from build123d import *

# Parameters (mm, degrees)
F1_DEPTH  = 459.486
F2_T      = -0.762
F5_D      = 5.2197
F5_DEPTH  = 0.762
F5_TIP    = 1.5681560866
F6_D      = 5.2197
F8_D      = 49.022
F10_D     = 17.4625
F13_D     = 5.2197
F13_DEPTH = 0.762
F13_TIP   = 1.5681560866


# Not quite as in the source:
# - a length typed as a fraction of an inch, garbled in the dataset ("3 / 203.2 mm" for 3/8 in), is restored


with BuildPart() as f1:
    # F0 (on Top) → F1 (new body)
    with BuildSketch(Plane.XY):
        Polygon((0, 360.045), (-512.445, 360.045), (-512.445, -360.045), (0, -360.045), (0, 0), align=None)
        Polygon((512.445, 360.045), (0, 360.045), (0, 0), (0, -360.045), (512.445, -360.045), align=None)
    extrude(amount=F1_DEPTH)

    # F2
    f2_openings = [f1.faces().sort_by_distance(p)[0] for p in [
        (0, 0, 459.486),
    ]]
    offset(amount=F2_T, openings=f2_openings)

    # F5
    with Locations(Plane.XZ.offset(360.045)):
        with Locations((-431.8, 415.036), (-215.9, 415.036), (0, 415.036), (215.9, 415.036), (431.8, 415.036)):
            Hole(F5_D / 2, depth=F5_DEPTH)
            with Locations((0, 0, -(F5_DEPTH + F5_TIP / 2))):  # 118° drill point
                Cone(0, F5_D / 2, F5_TIP, mode=Mode.SUBTRACT)

    # F6 (through all)
    with Locations(Plane.YZ.offset(512.445)):
        with Locations((-304.8, 415.036), (-101.6, 415.036), (101.6, 415.036), (304.8, 415.036)):
            Hole(F6_D / 2)

    # F8 (through all)
    with Locations(Plane.XY.offset(0.762)):
        with Locations((-371.475, -193.675)):
            Hole(F8_D / 2)

    # F10 (through all)
    with Locations(Plane.XY.offset(0.762)):
        with Locations((-485.775, 333.375), (-485.775, -333.375), (485.775, -333.375), (485.775, 333.375)):
            Hole(F10_D / 2)

    # F13
    with Locations(Plane(origin=(0, 360.045, 0), x_dir=(-1, 0, 0), z_dir=(0, 1, 0))):
        with Locations((-419.1, 445.1985), (-279.4, 445.1985), (-139.7, 445.1985), (0, 445.1985), (139.7, 445.1985), (279.4, 445.1985), (419.1, 445.1985)):
            Hole(F13_D / 2, depth=F13_DEPTH)
            with Locations((0, 0, -(F13_DEPTH + F13_TIP / 2))):  # 118° drill point
                Cone(0, F13_D / 2, F13_TIP, mode=Mode.SUBTRACT)


solid = f1.part
Work out the finished part from the listing and answer in its coordinate system (mm). A direction names the side the tool comes from. Round coordinates to 2 decimals unless told otherwise and drop trailing zeros. Loops run counter-clockwise (first coordinate to the right, second up) from the corner with the lowest first, then second, coordinate; pieces in that order, holes last. Notation, with made-up numbers: (84, 74.25) - (89, 74.25) arc R23 cw to (89, 112.25) - close; hole circle Ø3 at (19.25, -2). An arc over 180 degrees is marked (long way). Use one line per item in the form item = value. Start each with the question number.
(1) Find section C-C on z = 190. Determine the outline of the cut face in (x, y) (3 decimals), and give its area (3 significant figures).
(2) Find section B-B on x = 32.5. Determine the outline of the cut face in (y, z) (3 decimals), and give its area (3 significant figures).
(3) Consider line 1 (X direction, y = 194.5, z = 76.5) (3 decimals); line 2 (Y direction, x = -450, z = 439.5) (3 decimals); line 3 (Z direction, x = 469, y = 317). Determine where each line is inside the solid, lowest interval first.
(4) Which of the six approach directions +Z, -Z, +X, -X, +Y, -Y give full straight-line access (tool end or side, diameter ignored) to faces 5 (the face through (7, 360.045, 227)), 6 (the face through (-511.683, 5, 227))?
(5) Determine the mould class of faces 1 (the face through (512.445, -5, 227)), 2 (the face through (-7, 5, 0)), 3 (the face through (-512.445, 5, 227)), 4 (the face through (-7, 5, 0.762)) for opening direction X: +X half, -X half, draft (parallel to the pull), parting line (faces both ways), or undercut.
(6) Find section A-A on y = 9. Determine the outline of the cut face in (x, z) (3 decimals).
(7) Flat-ended cylindrical pins translate along their axes: P1, Ø7, axis at y = -304.8, z = 415.036, coming from the +X side (3 decimals); P2, Ø22.5, axis at x = -485.775, y = 333.375, coming from the +Z side; P3, Ø3, axis at x = -215.9, z = 415.036, coming from the -Y side. Find the tip coordinate at first contact, or state that the pin passes through.
Answer list:
q1.outline = (-512.445, -360.045) - (512.445, -360.045) - (512.445, 360.045) - (-512.445, 360.045) - close; hole (-511.683, -359.283) - (511.683, -359.283) - (511.683, 359.283) - (-511.683, 359.283) - close
q1.area = 2,660 mm^2
q2.outline = (-360.045, 0) - (360.045, 0) - (360.045, 459.486) - (359.283, 459.486) - (359.283, 0.762) - (-359.283, 0.762) - (-359.283, 459.486) - (-360.045, 459.486) - close
q2.area = 1,250 mm^2
q3.line_1 = -512.445 to -511.683, 511.683 to 512.445
q3.line_2 = -360.045 to -359.283, 359.283 to 360.045
q3.line_3 = 0 to 0.76
q4.face_5 = +Z, -Z, +X, -X, +Y
q4.face_6 = +Z
q5.face_1 = +X half
q5.face_2 = draft
q5.face_3 = -X half
q5.face_4 = undercut
q6.outline = (-512.445, 0) - (512.445, 0) - (512.445, 459.486) - (511.683, 459.486) - (511.683, 0.762) - (-511.683, 0.762) - (-511.683, 459.486) - (-512.445, 459.486) - close
q7.P1 = 512.445
q7.P2 = 0.76
q7.P3 = 359.28
